The model under review builds one solid part; all positions refer to its coordinate system, in mm. A direction names the side the tool comes from. Coordinates: 2 decimals unless noted, no trailing zeros. Order: outer loops, then holes, each group sorted by start corner. A loop starts at its lowest first (then second) coordinate and runs counter-clockwise, first axis right, second up. Notation, with made-up numbers: M -1.75,-38.75 L 29.25,-38.75 A11 ccw 29.25,-21.75 Z; hole C 1.5,0.5 d11. An arc over 180 degrees is marked long. Answer in a Markdown table with one row per item.
Autodesk Inventor part; units mm, degrees
ref_plane "YZ Plane" through (0, 0, 0) normal (1, 0, 0) x (0, 1, 0)
ref_plane "XZ Plane" through (0, 0, 0) normal (0, 1, 0) x (-1, 0, 0)
ref_plane "XY Plane" through (0, 0, 0) normal (0, 0, 1) x (1, 0, 0)
sketch "Sketch4" plane through (0, 0, 0) normal (0, 1, 0) x (-1, 0, 0)
  line L0 (0, 0) -> (-88, 0)
  line L1 (-88, 0) -> (-88, -82)
  line L2 (-88, -82) -> (0, -82)
  line L3 (0, -82) -> (0, 0)
  line L4 (-2.25, -82.75) -> (-85.75, -82.75) construction
  line L5 (-85.75, -82.75) -> (-85.75, 0.75) construction
  line L6 (-85.75, 0.75) -> (-2.25, 0.75) construction
  line L7 (-2.25, 0.75) -> (-2.25, -82.75) construction
  circle A0 centre (-44, -79.75) radius 1.6 construction
  circle A1 centre (-82.75, -41) radius 1.6 construction
  circle A2 centre (-5.25, -41) radius 1.6 construction
  circle A3 centre (-44, -2.25) radius 1.6 construction
  arc A4 (-42.0157, -82) -> (-45.9843, -82) centre (-44, -79.75) ccw
  circle A5 centre (-5.25, -41) radius 3
  arc A6 (-45.9843, 0) -> (-42.0157, 0) centre (-44, -2.25) ccw
  circle A7 centre (-82.75, -41) radius 3
  circle A8 centre (-3, -79) radius 1.5 construction
  circle A9 centre (-3, -3) radius 1.5 construction
  circle A10 centre (-85, -3) radius 1.5 construction
  circle A11 centre (-85, -79) radius 1.5 construction
  circle A12 centre (-3, -3) radius 3
  circle A13 centre (-85, -3) radius 3
  circle A14 centre (-85, -79) radius 3
  circle A15 centre (-3, -79) radius 3
  line L8 (-6, -3) -> (-41.0953, -3)
  line L9 (-46.9047, -3) -> (-82, -3)
  line L10 (-84, -76.1716) -> (-84, -43.7272)
  line L11 (-46.9047, -79) -> (-82, -79)
  line L12 (-5.2437, -79) -> (-41.0953, -79)
  line L13 (-4, -76.1716) -> (-4, -43.7272)
  line L14 (-4, -5.8284) -> (-4, -38.2728)
  line L15 (-84, -38.2728) -> (-84, -5.8284)
  point P0 (-3, -82)
  point P1 (0, -79)
  point P2 (0, -3)
  point P3 (-3, 0)
  point P4 (-85, 0)
  point P5 (-88, -3)
  point P6 (-88, -79)
  point P7 (-85, -82)
  point P8 (-6, -79)
  dimension "d40" = 88
  dimension "d41" = 82
  dimension "d42" = 83.5
  dimension "d43" = 2.25
  dimension "d44" = 0.75
  dimension "d45" = 3.2
  dimension "d47" = 3
  dimension "d48" = 3
  dimension "d49" = 3
  dimension "d50" = 3
  dimension "d51" = 41
  dimension "d52" = 44
  dimension "d53" = 6
  dimension "d54" = 3
  dimension "d55" = 3
  dimension "d56" = 3
  dimension "d57" = 3
  dimension "d58" = 3
  dimension "d59" = 6
  dimension "d60" = 3
  dimension "d61" = 3
  dimension "d62" = 4
  dimension "d63" = 4
extrude "Extrusion2" add sketch "Sketch4" along normal blind 5 contours A6 L0 | L0 A12 L8 A6 | A6 L9 A13 L0 | A12 | A13 | L3 A15 L13 A5 L14 A12 | A13 L15 A7 L10 A14 L1 | A15 | A14 | L2 A4 L12 A15 | A5 | A7 | A14 L11 A4 L2 | L2 A4
sketch "Sketch5" plane through (0, 5, 0) normal (0, 1, 0) x (1, 0, 0)
  arc A0 (84, 43.7272) -> (84, 38.2728) centre (82.75, 41) ccw
  arc A1 (41.0953, 79) -> (46.9047, 79) centre (44, 79.75) ccw
  arc A2 (46.9047, 3) -> (41.0953, 3) centre (44, 2.25) ccw
  arc A3 (4, 38.2728) -> (4, 43.7272) centre (5.25, 41) ccw
  point P0 (0, 0)
hole "Hole3" at (44, 5, -79.75) at (82.75, 5, -41) at (44, 5, -2.25) at (5.25, 5, -41) direction (0, -1, 0) diameter 2.459 end through all
sketch "Sketch6" plane through (0, 5, 0) normal (0, 1, 0) x (1, 0, 0)
  arc A0 (4, 76.1716) -> (6, 79) centre (3, 79) ccw
  arc A1 (6, 3) -> (4, 5.8284) centre (3, 3) ccw
  arc A2 (82, 79) -> (84, 76.1716) centre (85, 79) ccw
  arc A3 (84, 5.8284) -> (82, 3) centre (85, 3) ccw
  point P0 (0, 0)
hole "Hole4" at (85, 5, -79) at (85, 5, -3) at (3, 5, -3) at (3, 5, -79) direction (0, -1, 0) diameter 3.2 end through all
fillet "Fillet2" radius 3 16 edges at (41.0953, 2.5, -79) (46.9047, 2.5, -79) (6, 2.5, -79) (4, 2.5, -76.1716) (4, 2.5, -43.7272) (4, 2.5, -38.2728) (82, 2.5, -79) (84, 2.5, -76.1716) (84, 2.5, -38.2728) (84, 2.5, -43.7272) (82, 2.5, -3) (84, 2.5, -5.8284) (41.0953, 2.5, -3) (46.9047, 2.5, -3) (6, 2.5, -3) (4, 2.5, -5.8284)
equation "\"d43\" = -0.5 * d42 + 0.5 * d40"
equation "\"d44\" = -0.5 * d41 + 0.5 * d42"
equation "\"d48\" = d47"
equation "\"d50\" = d49"
equation "\"d51\" = 0.5 * d41"
equation "\"d52\" = 0.5 * d40"
properties part number "ElectronicsBayMount" material "Aluminum 6061"
(1) Take a section at B-B (z = -62). Write out the cut boundary in (x, y), then the cut area to 3 significant figures.
Report:
| item | result |
|---|---|
| outline | M 0,0 L 4,0 L 4,5 L 0,5 Z; M 84,0 L 88,0 L 88,5 L 84,5 Z |
| area | 40.0 mm^2 |
(2) Take a section at C-C (z = -41). Write out the cut boundary in (x, y).
Report:
| item | result |
|---|---|
| outline | M 0,0 L 4.02,0 L 4.02,5 L 0,5 Z; M 6.48,0 L 8.25,0 L 8.25,5 L 6.48,5 Z; M 79.75,0 L 81.52,0 L 81.52,5 L 79.75,5 Z; M 83.98,0 L 88,0 L 88,5 L 83.98,5 Z |
(3) Take a section at D-D (y = 1.75). State how many separate pieces and enclosed holes the cut face has, then the cut area to 3 significant figures.
Report:
| item | result |
|---|---|
| separate pieces | 1 |
| enclosed holes | 9 |
| area | 1,170 mm^2 |
(4) Take a section at A-A (x = 44). Write out the cut boundary in (y, z).
Report:
| item | result |
|---|---|
| outline | M 0,-82 L 5,-82 L 5,-80.98 L 0,-80.98 Z; M 0,-78.52 L 5,-78.52 L 5,-76.75 L 0,-76.75 Z; M 0,-5.25 L 5,-5.25 L 5,-3.48 L 0,-3.48 Z; M 0,-1.02 L 5,-1.02 L 5,0 L 0,0 Z |
(5) The part is to be moulded in two halves that separate along Z. For faces 1 (the cylindrical face through (0.86, 2.46, -81.1)), 2 (the flat face through (88, 2, -40)), 3 (the cylindrical face through (87.14, 2.46, -0.9)), 4 (the cylindrical face through (83.414, 2.465, -3.208)), say which applies: +Z half, -Z half, draft (parallel to the pull), parting line (faces both ways), or undercut.
Report:
| item | result |
|---|---|
| face 1 | -Z half |
| face 2 | draft |
| face 3 | +Z half |
| face 4 | undercut |
(6) Insertion check: P1, Ø2, axis at x = 44, z = -2.25, coming from the +Y side. The pin has a flat end and moves straight along its axis. Give the tip position at first contact, or say it passes through.
Report:
| item | result |
|---|---|
| P1 | through |
(7) To check wall thickness, follow line 1 (Z direction, x = 85, y = 3.8); line 2 (X direction, y = 1.8, z = -70.5); line 3 (Z direction, x = 68, y = 0.95). State the ranges of each line that lie inside material, in increasing order. Write a range as [from, to].
Report:
| item | result |
|---|---|
| line 1 | [-82, -80.6], [-77.4, -4.6], [-1.4, 0] |
| line 2 | [0, 4], [84, 88] |
| line 3 | [-82, -79], [-3, 0] |
(8) Machinability: for faces 5 (the flat face through (64, 2, -3)), 6 (the flat face through (0, 2, -42)), which of the approach directions +Z, -Z, +X, -X, +Y, -Y give a long, thin tool a straight path to every point of the face, cutting with its end or side? Answer none if there is none.
Report:
| item | result |
|---|---|
| face 5 | +Y, -Y |
| face 6 | +Z, -Z, -X, +Y, -Y |
